The listing builds one solid part. Answer for the finished solid, in the listing's coordinates (mm). Coordinates: 2 decimals unless noted, no trailing zeros. Order: outer loops, then holes, each group sorted by start corner. A loop starts at its lowest first (then second) coordinate and runs counter-clockwise, first axis right, second up. Notation, with made-up numbers: (-17, 74.5) -> (26, 74.5) arc R7 cw to (26, 81.5) -> close; hole circle Ø5 at (27.25, -22). An arc over 180 degrees is marked (long way). Return JSON: item names as keys, results as strings.
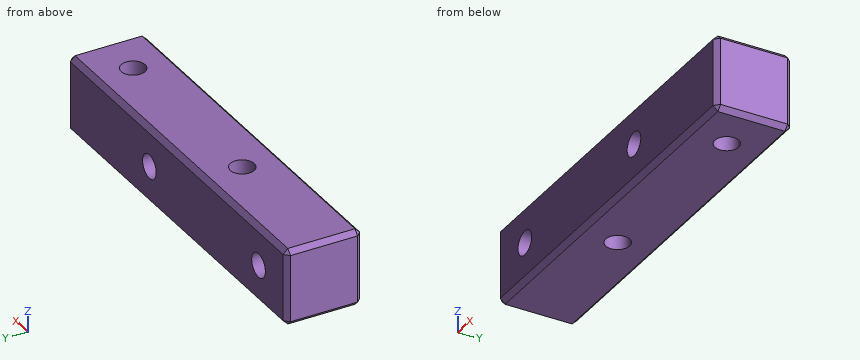
from build123d import *

# Parameters (mm, degrees)
SKETCH_2_W         = 40
SKETCH_2_H         = 8
SKETCH_2_R         = 0.5
EXTRUDE_1_DEPTH    = 4
HOLE_WIZARD_M3_1_D = 2.5
HOLE_WIZARD_M3_2_D = 2.5
CHAMFER_1_SIZE     = 0.5


with BuildPart() as part:
    # 草图2 → 凸台-拉伸1 (new body, symmetric)
    with BuildSketch(Plane.XY):
        with Locations((-15, 0)):
            Rectangle(SKETCH_2_W, SKETCH_2_H)
        with Locations((-20, 0)):
            Circle(SKETCH_2_R, mode=Mode.SUBTRACT)
        Circle(SKETCH_2_R, mode=Mode.SUBTRACT)
    extrude(amount=EXTRUDE_1_DEPTH, both=True)

    # M3 螺纹孔1 (through all)
    with Locations(Plane.XY.offset(4)):
        with Locations((0, 0), (-20, 0)):
            Hole(HOLE_WIZARD_M3_1_D / 2)

    # M3 螺纹孔2 (through all)
    with Locations(Plane(origin=(0, 4, 0), x_dir=(1, 0, 0), z_dir=(0, 1, 0))):
        with Locations((-10, 0), (-30, 0)):
            Hole(HOLE_WIZARD_M3_2_D / 2)

    # 倒角1
    chamfer_1_edges = [part.edges().sort_by_distance(p)[0] for p in [
        (-15, -4, 4),
        (5, 0, 4),
        (-15, 4, 4),
        (5, 0, -4),
        (-15, -4, -4),
        (-35, 0, -4),
        (-15, 4, -4),
        (-35, 0, 4),
        (5, 4, 0),
        (5, -4, 0),
        (-35, -4, 0),
        (-35, 4, 0),
    ]]
    chamfer(chamfer_1_edges, length=CHAMFER_1_SIZE)


solid = part.part
1. The part is cut by section B-B on y = 0. Give the vertices of the cut face in (x, z), and give its area (3 significant figures).
Answer block:
{"outline": "(-35, -3.5) -> (-34.5, -4) -> (-21.25, -4) -> (-21.25, 4) -> (-34.5, 4) -> (-35, 3.5) -> close; (-18.75, -4) -> (-1.25, -4) -> (-1.25, 4) -> (-18.75, 4) -> close; (1.25, -4) -> (4.5, -4) -> (5, -3.5) -> (5, 3.5) -> (4.5, 4) -> (1.25, 4) -> close; hole circle Ø2.5 at (-30, 0); hole circle Ø2.5 at (-10, 0)", "area": "270 mm2"}
2. This flat-tipped pin is pushed along its axis until it touches: pin 1 Ø4 at (x, y) = (0, 0) entering from +Z. Where does it stop, or does it pass through?
Answer block:
{"pin 1": "stops at z = 4"}
3. The part is cut by section A-A on z = 0. Give the vertices of the cut face in (x, y).
Answer block:
{"outline": "(-35, -3.5) -> (-34.5, -4) -> (-31.25, -4) -> (-31.25, 4) -> (-34.5, 4) -> (-35, 3.5) -> close; (-28.75, -4) -> (-11.25, -4) -> (-11.25, 4) -> (-28.75, 4) -> close; (-8.75, -4) -> (4.5, -4) -> (5, -3.5) -> (5, 3.5) -> (4.5, 4) -> (-8.75, 4) -> close; hole circle Ø2.5 at (-20, 0); hole circle Ø2.5 at (0, 0)"}
4. The part is cut by section D-D on y = -1.75. Give the vertices of the cut face in (x, z).
Answer block:
{"outline": "(-35, -3.5) -> (-34.5, -4) -> (4.5, -4) -> (5, -3.5) -> (5, 3.5) -> (4.5, 4) -> (-34.5, 4) -> (-35, 3.5) -> close; hole circle Ø2.5 at (-30, 0); hole circle Ø2.5 at (-10, 0)"}
5. Consider line 1 (Z direction, x = -30, y = 0); line 2 (X direction, y = -2.25, z = 0.25); line 3 (X direction, y = 3.5, z = -0.5). Determine where each line is inside the solid, lowest interval first. Write a range as from..to.
Answer block:
{"line 1": "z = -4..-1.25, 1.25..4", "line 2": "x = -35..-31.22, -28.78..-11.22, -8.78..5", "line 3": "x = -35..-31.15, -28.85..-11.15, -8.85..5"}
6. The part is cut by section C-C on z = 2.5. Give the vertices of the cut face in (x, y).
Answer block:
{"outline": "(-35, -3.5) -> (-34.5, -4) -> (4.5, -4) -> (5, -3.5) -> (5, 3.5) -> (4.5, 4) -> (-34.5, 4) -> (-35, 3.5) -> close; hole circle Ø2.5 at (-20, 0); hole circle Ø2.5 at (0, 0)"}
